```python
from build123d import *

# Parameters (mm, degrees)
BOSS_EXTRUDE1_DEPTH = 10
FILLET3_R           = 0.2
FILLET4_R           = 1


with BuildPart() as part:
    # Sketch1 → Boss-Extrude1 (new body)
    with BuildSketch(Plane.XY):
        Polygon((-48, 2.11152184), (-48, 5), (7, 5), (7, -10), (0, -10), (0, 0), (-16.5, 0), (-16.5, -20), (-21.5, -20), (-21.5, 0), (-30.5, 3), (-36.5, 3), (-35.093099913, 0.5), (-37.093099913, 0.5), (-38, 2.11152184), align=None)
    extrude(amount=BOSS_EXTRUDE1_DEPTH)

    # Fillet3
    fillet3_edges = [part.edges().sort_by_distance(p)[0] for p in [
        (-36.5, 3, 5),
        (-35.093099913, 0.5, 5),
        (-38, 2.11152184, 5),
        (-21.5, 0, 5),
        (-30.5, 3, 5),
    ]]
    fillet(fillet3_edges, radius=FILLET3_R)

    # Fillet4
    fillet4_edges = [part.edges().sort_by_distance(p)[0] for p in [
        (-48, 3.55576092, 0),
        (-48, 2.11152184, 5),
        (-48, 5, 5),
        (7, 5, 5),
        (0, 0, 5),
        (-16.5, 0, 5),
        (-48, 3.55576092, 10),
    ]]
    fillet(fillet4_edges, radius=FILLET4_R)


solid = part.part
```
Here's how the part is built. I have some questions about the finished solid (model axes, mm). A direction names the side the tool comes from. Coordinates: 2 decimals unless noted, no trailing zeros. Order: outer loops, then holes, each group sorted by start corner. A loop starts at its lowest first (then second) coordinate and runs counter-clockwise, first axis right, second up. Notation, with made-up numbers: M -24.5,5.25 L 30.5,5.25 A15 ccw 30.5,23.25 Z; hole C 50.5,-20.5 d1. An arc over 180 degrees is marked long. Answer as a JSON object with one key per item and string values. Group by question number.
(1) Suppose I cut it at B-B, the plane z = 3. Please give me the cut outline in (x, y).
(2) Suppose I cut it at A-A, the plane y = -9.5. Please give me the cut outline in (x, z).
(3) I need wall thicknesses on probe 1 along X at (y, z) = (-3, 7.75); probe 2 along Y at (x, z) = (-36, 5.5); probe 3 along Y at (x, z) = (-0.5, 3.5). Which ranges of each line are inside material? Lowest first, please.
(4) Which directions (+Z, -Z, +X, -X, +Y, -Y) give clear straight access to the entire face, cutting with the end or side of a thin tool? Please do faces 1 (the face through (-47.6, 3.6, 0.2)), 2 (the face through (0, -6, 5)), 3 (the face through (-36, 0.5, 5)).
(5) Suppose I cut it at D-D, the plane y = -14.5. Please give me the cut outline in (x, z).
(6) For pin 1 (1 mm diameter, centred on x = -37, z = 4.5, fed in from -Y); pin 2 (5 mm diameter, centred on x = -9.5, z = 2.5, fed in from -Y); pin 3 (5 mm diameter, centred on y = -14, z = 6.5, fed in from +X), each with a flat end and sliding along its axis, tell me the tip position at first contact or that it passes through.
(7) Suppose I cut it at C-C, the plane x = -3.5. Please give me the cut outline in (y, z).
(8) If we mould it in two halves opening along X, with no side actions, what happens to faces 4 (the face through (-21.5, -10, 5)), 5 (the face through (-12, 1, 0)), 6 (the face through (-35.8, 1.76, 4.93))? For each: released by +X, released by -X, zero draft, split by the parting line, or undercut.
Values found:
{
 "1": {"outline": "M -48,3.11 A1 ccw -47,2.11 L -38.12,2.11 A0.2 cw -37.94,2.01 L -37.09,0.5 L -35.44,0.5 A0.2 ccw -35.26,0.8 L -36.33,2.7 A0.2 cw -36.16,3 L -30.53,3 A0.2 cw -30.47,2.99 L -21.64,0.05 A0.2 cw -21.5,-0.14 L -21.5,-20 L -16.5,-20 L -16.5,-1 A1 cw -15.5,0 L -1,0 A1 cw 0,-1 L 0,-10 L 7,-10 L 7,4 A1 ccw 6,5 L -47,5 A1 ccw -48,4 Z"},
 "2": {"outline": "M -21.5,0 L -16.5,0 L -16.5,10 L -21.5,10 Z; M 0,0 L 7,0 L 7,10 L 0,10 Z"},
 "3": {"probe 1": "x = -21.5 to -16.5, 0 to 7", "probe 2": "y = 0.5 to 2.11, 3 to 5", "probe 3": "y = -0.13 to 5"},
 "4": {"face 1": "-Z, -X, +Y, -Y", "face 2": "+Z, -Z, -Y", "face 3": "+Z, -Z, -X, -Y"},
 "5": {"outline": "M -21.5,0 L -16.5,0 L -16.5,10 L -21.5,10 Z"},
 "6": {"pin 1": "stops at y = 0.5", "pin 2": "stops at y = 0", "pin 3": "stops at x = -16.5"},
 "7": {"outline": "M 0,0 L 5,0 L 5,10 L 0,10 Z"},
 "8": {"face 4": "released by -X", "face 5": "zero draft", "face 6": "undercut"}
}
